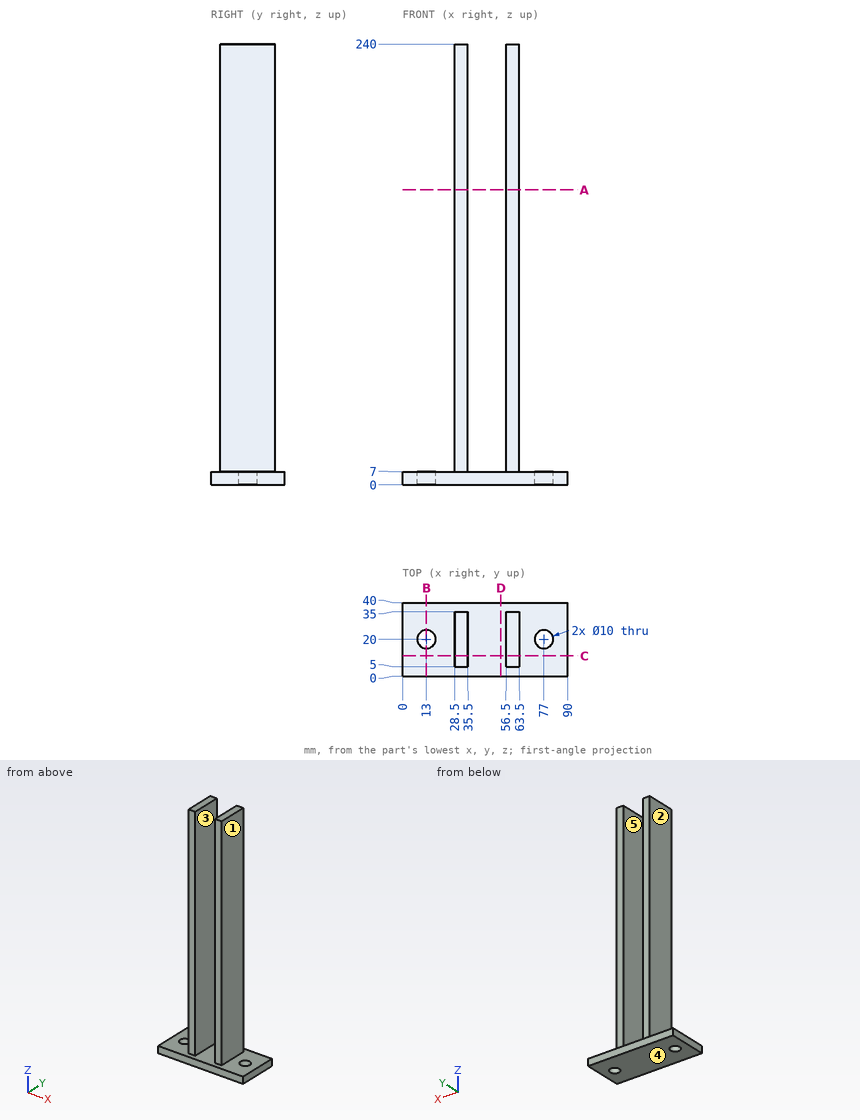
Design review of the part shown in the three views and the two pictorial views. Dimensions are in mm from the part's minimum x, y and z. A direction names the side the tool comes from. Round coordinates to 2 decimals unless told otherwise and drop trailing zeros. Write each loop counter-clockwise with the first axis right and the second up, starting at its lowest first coordinate (ties: lowest second). Pieces come first, ordered by that corner, then holes. Notation, with made-up numbers: (74.25, 87) -> (79.25, 87) arc R22 cw to (79.25, 120) -> close; hole circle Ø8 at (50, -15). An arc over 180 degrees is marked (long way). Answer as a JSON object with one key per item and string values.
1. The part is to be moulded in two halves that separate along X. For the marked faces 1, 2 and 3, say which applies: pulls with the +X half, pulls with the -X half, needs draft (parallel to the pull), parting line crosses it, or undercut.
Results found:
{"face 1": "pulls with the +X half", "face 2": "pulls with the -X half", "face 3": "undercut"}
2. Clearance check with flat-ended pins moving along their axes: pin 1 (15 mm diameter, centred on y = 20, z = 137, fed in from +X); pin 2 (5.5 mm diameter, centred on x = 60.5, z = 181.5, fed in from -Y); pin 3 (24 mm diameter, centred on y = 21.5, z = 98.5, fed in from -X); pin 4 (8 mm diameter, centred on x = 77, y = 20, fed in from -Z). State where each tip first meets the part, or that it passes through.
Results found:
{"pin 1": "stops at x = 63.5", "pin 2": "stops at y = 5", "pin 3": "stops at x = 28.5", "pin 4": "passes through"}
3. We need section A-A on z = 160.5. State the section outline as (x, y) points.
Results found:
{"outline": "(28.5, 5) -> (35.5, 5) -> (35.5, 35) -> (28.5, 35) -> close; (56.5, 5) -> (63.5, 5) -> (63.5, 35) -> (56.5, 35) -> close"}
4. Machinability: for the marked faces 4 and 5, which of the approach directions +Z, -Z, +X, -X, +Y, -Y give a long, thin tool a straight path to every point of the face, cutting with its end or side? Answer none if there is none.
Results found:
{"face 4": "-Z, +X, -X, +Y, -Y", "face 5": "+Z, +Y, -Y"}
5. We need section B-B on x = 13. State the section outline as (y, z) points, and give its area (3 significant figures).
Results found:
{"outline": "(0, 0) -> (15, 0) -> (15, 7) -> (0, 7) -> close; (25, 0) -> (40, 0) -> (40, 7) -> (25, 7) -> close", "area": "210 mm^2"}
6. To check wall thickness, follow line 1 along X through (y, z) = (20, 4); line 2 along X through (y, z) = (34, 184.5); line 3 along Y through (x, z) = (77, 5). State the ranges of each line that lie inside material, in increasing order.
Results found:
{"line 1": "x = 0 to 8, 18 to 72, 82 to 90", "line 2": "x = 28.5 to 35.5, 56.5 to 63.5", "line 3": "y = 0 to 15, 25 to 40"}
7. We need section C-C on y = 11. State the section outline as (x, z) points.
Results found:
{"outline": "(0, 0) -> (90, 0) -> (90, 7) -> (63.5, 7) -> (63.5, 240) -> (56.5, 240) -> (56.5, 7) -> (35.5, 7) -> (35.5, 240) -> (28.5, 240) -> (28.5, 7) -> (0, 7) -> close"}
8. We need section D-D on x = 53.5. State the section outline as (y, z) points, and give its area (3 significant figures).
Results found:
{"outline": "(0, 0) -> (40, 0) -> (40, 7) -> (0, 7) -> close", "area": "280 mm^2"}
